from build123d import *

# Parameters (mm, degrees)
F0_W     = 150
F0_H     = 40
F1_DEPTH = 10
F3_DEPTH = 7
F4_W     = 44.4098300563
F4_H     = 3
F5_DEPTH = 4
F6_R     = 5.08
F7_W     = 20.7056045532
F7_H     = 40
F7_W_2   = 21.5539429337
F8_DEPTH = 25.4


with BuildPart() as f1:
    # F0 (on Top) → F1 (new body)
    with BuildSketch(Plane.XY):
        with Locations((-27.5264725089, -48.8547566533)):
            Rectangle(F0_W, F0_H)
    extrude(amount=F1_DEPTH)

    # F2 (on face) → F3 (cut)
    with BuildSketch(Plane.XY.offset(10)):
        with BuildLine():
            Line((-77.5264725089, -43.8547566533), (-77.5264725089, -48.8547566533))
            Line((-77.5264725089, -48.8547566533), (-77.5264725089, -53.8547566533))
            Line((-77.5264725089, -53.8547566533), (-33.1166424527, -53.8547566533))
            ThreePointArc((-33.1166424527, -53.8547566533), (-27.5264725089, -56.3547566533), (-21.9363025652, -53.8547566533))
            Line((-21.9363025652, -53.8547566533), (22.4735274911, -53.8547566533))
            Line((22.4735274911, -53.8547566533), (22.4735274911, -48.8547566533))
            Line((22.4735274911, -48.8547566533), (22.4735274911, -43.8547566533))
            Line((22.4735274911, -43.8547566533), (-21.9363025652, -43.8547566533))
            ThreePointArc((-21.9363025652, -43.8547566533), (-27.5264725089, -41.3547566533), (-33.1166424527, -43.8547566533))
            Line((-33.1166424527, -43.8547566533), (-77.5264725089, -43.8547566533))
        make_face()
        with BuildLine():
            ThreePointArc((-25.0264725089, -48.8547566533), (-27.5264725089, -51.3547566533), (-30.0264725089, -48.8547566533))
            ThreePointArc((-30.0264725089, -48.8547566533), (-27.5264725089, -46.3547566533), (-25.0264725089, -48.8547566533))
        make_face(mode=Mode.SUBTRACT)
    extrude(amount=-F3_DEPTH, mode=Mode.SUBTRACT)

    # F4 (on face) → F5 (join)
    with BuildSketch(Plane.XY.offset(3)):
        with Locations((-55.3215574808, -45.3547566533)):
            Rectangle(F4_W, F4_H)
        with Locations((-55.3215574808, -52.3547566533)):
            Rectangle(F4_W, F4_H)
        with Locations((0.268612463, -52.3547566533)):
            Rectangle(F4_W, F4_H)
        with Locations((0.268612463, -45.3547566533)):
            Rectangle(F4_W, F4_H)
    extrude(amount=F5_DEPTH)

    # F6
    f6_edges = [f1.edges().sort_by_distance(p)[0] for p in [
        (-77.526473, -48.854757, 3),
        (22.473527, -48.854757, 3),
    ]]
    fillet(f6_edges, radius=F6_R)

    # F7 (on face) → F8 (cut)
    with BuildSketch(Plane.XY.offset(10)):
        with Locations((-92.1736702323, -48.8547566533)):
            Rectangle(F7_W, F7_H)
        with Locations((36.6965560243, -48.8547566533)):
            Rectangle(F7_W_2, F7_H)
    extrude(amount=-F8_DEPTH, mode=Mode.SUBTRACT)


solid = f1.part
Source: CAD feature listing. Evaluate the final solid. Frame: model axes, mm. A direction names the side the tool comes from. Round coordinates to 2 decimals unless told otherwise and drop trailing zeros. Write each loop counter-clockwise with the first axis right and the second up, starting at its lowest first coordinate (ties: lowest second). Pieces come first, ordered by that corner, then holes. Notation, with made-up numbers: M 38.5,80 L 91.5,80 A24 cw 91.5,113 Z; hole C 82.5,7.5 d6. An arc over 180 degrees is marked long. One line per item, written item: value. Start each with the question number.
Item 1: Set-up query: faces 5 (the cylindrical face through (-76.64, -48.92, 5.21)), 6 (the flat face through (-29, -57, 10)). Return all of +Z, -Z, +X, -X, +Y, -Y with unobstructed straight access to the full face (end or side cutting, diameter ignored); none if empty.
Item 2: Pin query (flat end, axial travel): pin 1 (1.5 mm diameter, centred on x = 2, y = -46, fed in from +Z). Return the tip coordinate at first contact, or that it passes through.
Item 3: Section query B-B (x = 1). Return the cut outline in (y, z), plus the area to 3 significant figures.
Item 4: Ray query, L1, parallel to Y at x = 7, z = 4.25; L2, parallel to Y at x = -55.5, z = 8.25; L3, parallel to Z at x = 15.5, y = -44. Return the intervals inside material, ascending. Write a range as from..to.
Item 5: Mould query, pull axis X, two halves, no side actions, for faces 1 (the flat face through (-56, -53.855, 9)), 2 (the flat face through (-81.821, -49, 5)), 3 (the flat face through (-28, -49, 10)), 4 (the flat face through (0, -53.855, 9)). Classes: pulls with the +X half, pulls with the -X half, needs draft (parallel to the pull), parting line crosses it, or undercut.
Item 6: Section query A-A (z = 4). Return the cut outline in (x, y).
Result set:
1. face 5: +Z
1. face 6: +Z, +X, -X, +Y, -Y
2. pin 1: stops at z = 7
3. outline: M -68.85,0 L -28.85,0 L -28.85,10 L -43.85,10 L -43.85,7 L -46.85,7 L -46.85,3 L -50.85,3 L -50.85,7 L -53.85,7 L -53.85,10 L -68.85,10 Z
3. area: 354 mm²
4. L1: y = -68.85..-50.85, -46.85..-28.85
4. L2: y = -68.85..-53.85, -43.85..-28.85
4. L3: z = 0..7
5. face 1: undercut
5. face 2: pulls with the -X half
5. face 3: needs draft
5. face 4: undercut
6. outline: M -81.82,-68.85 L 25.92,-68.85 L 25.92,-28.85 L -81.82,-28.85 Z; C -27.53,-48.85 d5; hole M -75.47,-50.85 L -33.12,-50.85 L -33.12,-53.85 A7.5 ccw -21.94,-53.85 L -21.94,-50.85 L 20.42,-50.85 L 20.42,-46.85 L -21.94,-46.85 L -21.94,-43.85 A7.5 ccw -33.12,-43.85 L -33.12,-46.85 L -75.47,-46.85 Z
